Geometry check sheet. Reference: the model listing, model coordinates, mm. Coordinates: 2 decimals unless noted, no trailing zeros. Loops run counter-clockwise (first coordinate to the right, second up) from the corner with the lowest first, then second, coordinate; pieces in that order, holes last. Notation, with made-up numbers: (-17, -25) - (-6, -25) arc R11 ccw to (-6, -20) - close; hole circle Ø1 at (-11, 16). An arc over 180 degrees is marked (long way). Write each question's results on one line, items separated by ' | '. Start each with the question number.
(1) Sectioned sample at D-D (x = -10). State how many separate pieces and enclosed holes the cut face has, plus the area to 3 significant figures.
(2) Go/stop test with flat-tipped pins: pin 1 Ø8 at (y, z) = (-14.5, 0.5) entering from -X; pin 2 Ø12 at (y, z) = (-87, 14) entering from +X; pin 3 Ø5 at (y, z) = (-10, 1) entering from +X. Record where each tip stops, or that it passes through.
(3) Mould release check, pull along Y, two halves, no side actions. Record for faces 1 (the face through (-3.05, -103.917, 6.135)), 2 (the face through (-4, -48, 29.799)), 3 (the face through (-4.622, -68.087, -0.775)): pulls with the +Y half, pulls with the -Y half, needs draft (parallel to the pull), parting line crosses it, or undercut.
(4) Material ranges on probe 1 along Z at (x, y) = (-10, -55); probe 2 along Z at (x, y) = (-15, -39); probe 3 along X at (y, z) = (-9, -4.5), recorded low to high.
(5) Sectioned sample at B-B (z = -8). Enter the section's corners in (x, y).
(6) Sectioned sample at A-A (z = 10.5). Enter the section's corners in (x, y).
(7) Sectioned sample at C-C (z = 16). Enter the section's corners in (x, y).
from build123d import *

# Parameters (mm, degrees)
F0_W      = 60
F0_H      = 48
F0_R      = 4.75
F1_DEPTH  = 108
F3_DEPTH  = 48
F5_DEPTH  = 48
F7_DEPTH  = 48
F9_DEPTH  = 48
F10_ANGLE = -15


with BuildPart() as f1:
    # F0 (on Front) → F1 (new body)
    with BuildSketch(Plane.XZ):
        with Locations((11.7113751173, 5.7986730486)):
            Rectangle(F0_W, F0_H)
        with Locations((0.7113751173, -2.2013269514)):
            Circle(F0_R, mode=Mode.SUBTRACT)
        with Locations((0.7113751173, 13.7986730486)):
            Circle(F0_R, mode=Mode.SUBTRACT)
    extrude(amount=F1_DEPTH)

    # F2 (on face) → F3 (cut)
    with BuildSketch(Plane(origin=(0, 0, -18.2013269514), x_dir=(1, 0, 0), z_dir=(0, 0, -1))):
        Polygon((10.7113751173, 0), (-18.2886248827, 108), (-18.2886248827, 0), align=None)
    extrude(amount=-F3_DEPTH, mode=Mode.SUBTRACT)

    # F4 (on face) → F5 (cut)
    with BuildSketch(Plane(origin=(0, 0, -18.2013269514), x_dir=(1, 0, 0), z_dir=(0, 0, -1))):
        Polygon((41.7113751173, 108), (41.7113751173, 3.724137931), (42.3088373496, 1.4991061694), (42.3088373496, 108), align=None)
        Polygon((41.7113751173, 108), (13.7113751173, 108), (41.7113751173, 3.724137931), align=None)
    extrude(amount=-F5_DEPTH, mode=Mode.SUBTRACT)

    # F6 (on face) → F7 (cut)
    with BuildSketch(Plane(origin=(0, 0, -18.2013269514), x_dir=(1, 0, 0), z_dir=(0, 0, -1))):
        Polygon((41.7113751173, 3.724137931), (10.7113751173, 0), (41.7113751173, 0), align=None)
    extrude(amount=-F7_DEPTH, mode=Mode.SUBTRACT)

    # F8 (on face) → F9 (cut)
    with BuildSketch(Plane(origin=(0, 0, -18.2013269514), x_dir=(1, 0, 0), z_dir=(0, 0, -1))):
        Polygon((40.559275957, 8.0147141144), (10.7113751173, 0), (42.3792054196, 1.2370457707), align=None)
    extrude(amount=-F9_DEPTH, mode=Mode.SUBTRACT)


with BuildPart() as f1_1:
    # F10: moved
    add(f1.part.rotate(Axis((-18.2886248827, -108, 5.7986730486), (0, 0, -1)), F10_ANGLE))


solid = f1_1.part
Outcome:
1) separate pieces: 1 | enclosed holes: 2 | area: 4,710 mm2
2) pin 1: stops at x = -18.24 | pin 2: stops at x = 12.63 | pin 3: stops at x = 12.67
3) face 1: pulls with the -Y half | face 2: needs draft | face 3: undercut
4) probe 1: z = -18.2 to -6.09, 1.69 to 9.91, 17.69 to 29.8 | probe 2: z = -18.2 to -6.49, 2.09 to 9.51, 18.09 to 29.8 | probe 3: x = -18.24 to 12.67
5) outline: (-18.29, -108) - (12.62, -99.72) - (12.68, 3.81) - (-18.23, 3.83) - close
6) outline: (-18.29, -108) - (-3.24, -103.97) - (-18.26, -47.91) - close; (-18.24, -21.56) - (3.37, -102.2) - (12.62, -99.72) - (12.68, 3.81) - (-18.23, 3.83) - close
7) outline: (-18.29, -108) - (-4, -104.17) - (-18.26, -50.97) - close; (-18.24, -18.5) - (4.13, -101.99) - (12.62, -99.72) - (12.68, 3.81) - (-18.23, 3.83) - close
